Part model, mm, in its own coordinate system. A direction names the side the tool comes from. Round coordinates to 2 decimals unless told otherwise and drop trailing zeros. Write each loop counter-clockwise with the first axis right and the second up, starting at its lowest first coordinate (ties: lowest second). Pieces come first, ordered by that corner, then holes. Notation, with made-up numbers: M 66.25,-25.75 L 98.25,-25.75 A30 cw 98.25,-1.75 Z; hole C 34,28.5 d8. An arc over 180 degrees is marked long. Answer as a JSON object with one key per item and string values. Group by question number.
1. Which spindle directions (+Z, -Z, +X, -X, +Y, -Y) get a long thin tool onto all of the face, cutting with end or side? Do faces 4 (the face through (4, 0, 2)), 5 (the face through (-1.225, -1.206, 3.131)). Say none if no direction does.
2. Band-saw the part on A-A, the plane y = 3.25. Write the cut outline in (x, z).
3. Band-saw the part on C-C, the plane z = 1. Write the cut outline in (x, y), plus the area to 3 significant figures.
4. Band-saw the part on B-B, the plane x = 4. Write the cut outline in (y, z).
5. Drill centre lines: line 1 (Y direction, x = 5, z = 0.5); line 2 (Y direction, x = 0.25, z = 1). Where is each one in solid material? Low to high. Write a range as from..to.
6. Drop flat-ended pins along their axis: pin 1 (3 mm diameter, centred on x = 3.5, z = 1, fed in from +Y); pin 2 (3 mm diameter, centred on y = 4, z = 3.5, fed in from +X). Give the stop position or say it passes through.
7. Two-plate mould, pull along Z, no slides. Class faces 1 (the face through (4, -1.588, 2)), 2 (the face through (-0.805, 1.957, 2.817)), 3 (the face through (0, 0, 6.35)): +Z half, -Z half, draft (parallel to the pull), parting line (faces both ways), or undercut.
8. Band-saw the part on D-D, the plane z = 1.75. Write the cut outline in (x, y), plus the area to 3 significant figures.
from build123d import *

# Parameters (mm, degrees)
BOSS_EXTRUDE1_DEPTH       = 6.35
F_4_CLEARANCE_HOLE1_D     = 3.302
F_4_CLEARANCE_HOLE1_DEPTH = 57.15
F_4_CLEARANCE_HOLE1_TIP   = 0.992020882
F_4_40_TAPPED_HOLE1_D     = 2.2606


with BuildPart() as part:
    # Sketch1 → Boss-Extrude1 (new body)
    with BuildSketch(Plane.XY):
        with BuildLine():
            Line((0, 1.27), (0, 7.1247))
            Line((0, 7.1247), (-1.5875, 7.1247))
            Line((-1.5875, 7.1247), (-1.5875, -0.3175))
            ThreePointArc((-1.5875, -0.3175), (-1.215525612, -1.215525612), (-0.3175, -1.5875))
            Line((-0.3175, -1.5875), (7.9375, -1.5875))
            Line((7.9375, -1.5875), (7.9375, 0))
            Line((7.9375, 0), (1.27, 0))
            ThreePointArc((1.27, 0), (0.371974388, 0.371974388), (0, 1.27))
        make_face()
    extrude(amount=BOSS_EXTRUDE1_DEPTH)

    # #4 Clearance Hole1
    with Locations(Plane(origin=(0, 0, 0), x_dir=(0, 0, -1), z_dir=(1, 0, 0))):
        with Locations((-3.175, 3.5687)):
            Hole(F_4_CLEARANCE_HOLE1_D / 2, depth=F_4_CLEARANCE_HOLE1_DEPTH)
            with Locations((0, 0, -(F_4_CLEARANCE_HOLE1_DEPTH + F_4_CLEARANCE_HOLE1_TIP / 2))):  # 118° drill point
                Cone(0, F_4_CLEARANCE_HOLE1_D / 2, F_4_CLEARANCE_HOLE1_TIP, mode=Mode.SUBTRACT)

    # #4-40 Tapped Hole1 (through all)
    with Locations(Plane(origin=(0, 0, 0), x_dir=(1, 0, 0), z_dir=(0, 1, 0))):
        with Locations((4.7625, -3.175)):
            Hole(F_4_40_TAPPED_HOLE1_D / 2)


solid = part.part
Worked answers:
{
 "1": {"face 4": "+Z, -Z, +X, +Y", "face 5": "+Z, -Z, -X, -Y"},
 "2": {"outline": "M -1.59,0 L 0,0 L 0,1.56 L -1.59,1.56 Z; M -1.59,4.79 L 0,4.79 L 0,6.35 L -1.59,6.35 Z"},
 "3": {"outline": "M -1.59,-0.32 A1.27 ccw -0.32,-1.59 L 7.94,-1.59 L 7.94,0 L 1.27,0 A1.27 cw 0,1.27 L 0,7.12 L -1.59,7.12 Z", "area": "26.4 mm^2"},
 "4": {"outline": "M -1.59,0 L 0,0 L 0,2.34 L -1.59,2.34 Z; M -1.59,4.01 L 0,4.01 L 0,6.35 L -1.59,6.35 Z"},
 "5": {"line 1": "y = -1.59..0", "line 2": "y = -1.59..0.51"},
 "6": {"pin 1": "stops at y = 0", "pin 2": "stops at x = 0"},
 "7": {"face 1": "draft", "face 2": "undercut", "face 3": "+Z half"},
 "8": {"outline": "M -1.59,-0.32 A1.27 ccw -0.32,-1.59 L 7.94,-1.59 L 7.94,0 L 1.27,0 A1.27 cw 0,1.27 L 0,2.73 L -1.59,2.73 Z; M -1.59,4.4 L 0,4.4 L 0,7.12 L -1.59,7.12 Z", "area": "23.8 mm^2"}
}
